Input: part model. Units: mm. Frame: model coordinates. Coordinates: 2 decimals unless noted, no trailing zeros. Write each loop counter-clockwise with the first axis right and the second up, starting at its lowest first coordinate (ties: lowest second). Pieces come first, ordered by that corner, then holes. Notation, with made-up numbers: (47.25, 49.5) -> (62.25, 49.5) arc R24 cw to (62.25, 84.5) -> close; hole circle Ø1 at (80, 37). An arc over 180 degrees is marked (long way). Use one line per item in the form item = value. Start each with the question number.
(1) Cut plane A-A on z = 4. Return the cut outline in (x, y) (3 decimals).
(2) Cut plane D-D on x = -30.5. Return the cut outline in (y, z) (3 decimals), plus the area to 3 significant figures.
(3) First-contact query: pin 1 (18.5 mm diameter, centred on x = 82.55, z = 51, fed in from +Y) (3 decimals); pin 2 (9.5 mm diameter, centred on x = -25.4, z = 51, fed in from +Y); pin 3 (0.7 mm diameter, centred on x = -36, y = 7, fed in from -Z) (3 decimals); pin 4 (2 mm diameter, centred on y = 8, z = 11, fed in from +X) (3 decimals). Flat tips, straight axial feed; report the tip coordinate or a pass-through.
(4) Cut plane B-B on x = 0. State how many separate pieces and enclosed holes the cut face has, plus the area to 3 significant figures.
(5) Ray query, line 1 along Z through (x, y) = (20.5, 3.5) (3 decimals); line 2 along Z through (x, y) = (20.5, 5) (3 decimals); line 3 along Z through (x, y) = (-70.5, 6) (3 decimals). Return the intervals inside material, ascending.
```python
from build123d import *

# Parameters (mm, degrees)
SKETCH1_W           = 203.2
SKETCH1_H           = 152.4
BOSS_EXTRUDE1_DEPTH = 9.525
SKETCH2_W           = 156.7
SKETCH2_H           = 89.1
CUT_EXTRUDE1_DEPTH  = 128.356686613
CHAMFER1_SIZE       = 2.54
SKETCH3_W           = 164.9
SKETCH3_H           = 100
CUT_EXTRUDE2_DEPTH  = 6.35
SKETCH4_R           = 7.9375
CUT_EXTRUDE3_DEPTH  = 128.356686613
CHAMFER2_SIZE       = 6.35


with BuildPart() as part:
    # Sketch1 → Boss-Extrude1 (new body)
    with BuildSketch(Plane(origin=(0, 0, 0), x_dir=(1, 0, 0), z_dir=(0, 1, 0))):
        Rectangle(SKETCH1_W, SKETCH1_H)
    extrude(amount=BOSS_EXTRUDE1_DEPTH)

    # Sketch2 → Cut-Extrude1 (cut, through all)
    with BuildSketch(Plane(origin=(0, 9.525, 0), x_dir=(1, 0, 0), z_dir=(0, 1, 0))):
        with Locations((0, 18.95)):
            Rectangle(SKETCH2_W, SKETCH2_H)
    extrude(amount=-CUT_EXTRUDE1_DEPTH, mode=Mode.SUBTRACT)

    # Chamfer1
    chamfer1_edges = [part.edges().sort_by_distance(p)[0] for p in [
        (78.35, 9.525, -18.95),
        (0, 9.525, -63.5),
        (-78.35, 9.525, -18.95),
        (0, 9.525, 25.6),
    ]]
    chamfer(chamfer1_edges, length=CHAMFER1_SIZE)

    # Sketch3 → Cut-Extrude2 (cut)
    with BuildSketch(Plane(origin=(-44.720558265, 0, -165.453357273), x_dir=(1, 0, 0), z_dir=(0, -1, 0))):
        with Locations((46.110558265, 148.383357273)):
            Rectangle(SKETCH3_W, SKETCH3_H)
    extrude(amount=-CUT_EXTRUDE2_DEPTH, mode=Mode.SUBTRACT)

    # Sketch4 → Cut-Extrude3 (cut, through all)
    with BuildSketch(Plane(origin=(0, 9.525, 0), x_dir=(1, 0, 0), z_dir=(0, 1, 0))):
        with Locations(Location((-50.8, -51, 0), (0, 0, 270))):
            Circle(SKETCH4_R)
        with Locations(Location((-25.4, -51, 0), (0, 0, 270))):
            Circle(SKETCH4_R)
        with Locations(Location((0, -51, 0), (0, 0, 270))):
            Circle(SKETCH4_R)
        with Locations(Location((25.4, -51, 0), (0, 0, 270))):
            Circle(SKETCH4_R)
        with Locations(Location((50.8, -51, 0), (0, 0, 270))):
            Circle(SKETCH4_R)
        with Locations(Location((82.55, -51, 0), (0, 0, 270))):
            Circle(SKETCH4_R)
    extrude(amount=-CUT_EXTRUDE3_DEPTH, mode=Mode.SUBTRACT)

    # Chamfer2
    chamfer2_edges = [part.edges().sort_by_distance(p)[0] for p in [
        (-101.6, 9.525, 0),
        (0, 9.525, 76.2),
        (101.6, 9.525, 0),
        (0, 9.525, -76.2),
    ]]
    chamfer(chamfer2_edges, length=CHAMFER2_SIZE)


solid = part.part
```
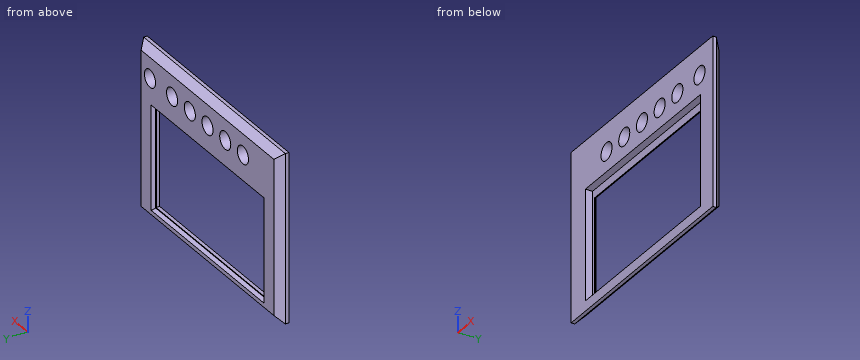
Values:
q1.outline = (-101.6, 0) -> (-81.06, 0) -> (-81.06, 6.35) -> (-78.35, 6.35) -> (-78.35, 6.985) -> (-80.89, 9.525) -> (-95.25, 9.525) -> (-101.6, 3.175) -> close; (78.35, 6.35) -> (83.84, 6.35) -> (83.84, 0) -> (101.6, 0) -> (101.6, 3.175) -> (95.25, 9.525) -> (80.89, 9.525) -> (78.35, 6.985) -> close
q2.outline = (0, -76.2) -> (3.175, -76.2) -> (9.525, -69.85) -> (9.525, -66.04) -> (6.985, -63.5) -> (6.35, -63.5) -> (6.35, -67.07) -> (0, -67.07) -> close; (0, 32.93) -> (6.35, 32.93) -> (6.35, 25.6) -> (6.985, 25.6) -> (9.525, 28.14) -> (9.525, 44.918) -> (0, 44.918) -> close; (0, 57.082) -> (9.525, 57.082) -> (9.525, 69.85) -> (3.175, 76.2) -> (0, 76.2) -> close
q2.area = 371 mm2
q3.pin_1 = 9.525
q3.pin_2 = through
q3.pin_3 = -72.725
q3.pin_4 = 97.775
q4.separate_pieces = 3
q4.enclosed_holes = 0
q4.area = 336 mm2
q5.line_1 = -75.875 to -67.07, 32.93 to 44.755, 57.245 to 75.875
q5.line_2 = -74.375 to -67.07, 32.93 to 44.755, 57.245 to 74.375
q5.line_3 = -73.375 to -67.07, 32.93 to 73.375
